from build123d import *

# Parameters (mm, degrees)
SKETCH2_W            = 38
SKETCH2_H            = 23.6
BOSS_EXTRUDE2_DEPTH  = 2.5
SKETCH3_W            = 35
SKETCH3_H            = 17.6
CUT_EXTRUDE2_DEPTH   = 2.5
SKETCH5_W            = 36.5
SKETCH5_H            = 2
SKETCH5_W_2          = 1.5
SKETCH5_H_2          = 19.6
BOSS_EXTRUDE3_DEPTH  = 26
SKETCH7_W            = 36.5
SKETCH7_H            = 2.5
BOSS_EXTRUDE5_DEPTH  = 1
SKETCH10_W           = 12.597499818
SKETCH10_H           = 2.5
SKETCH10_W_2         = 23.902500182
BOSS_EXTRUDE6_DEPTH  = 1
SKETCH11_W           = 2.5
SKETCH11_H           = 17.6
BOSS_EXTRUDE7_DEPTH  = 2
SKETCH15_W           = 30.589508609
SKETCH15_H           = 23.5
SKETCH15_W_2         = 3.8732763
CUT_EXTRUDE4_DEPTH   = 30
SKETCH16_W           = 3
SKETCH16_H           = 2.5
BOSS_EXTRUDE8_DEPTH  = 20
SKETCH17_W           = 3
SKETCH17_H           = 2.5
BOSS_EXTRUDE9_DEPTH  = 20
SKETCH19_W           = 5.5
SKETCH19_H           = 23.6
BOSS_EXTRUDE10_DEPTH = 16
SKETCH20_R           = 2.6
CUT_EXTRUDE6_DEPTH   = 30
SKETCH21_R           = 3.3
CUT_EXTRUDE7_DEPTH   = 0.8
SKETCH22_R           = 3.3
CUT_EXTRUDE8_DEPTH   = 0.8
FILLET1_R            = 5
FILLET3_R            = 5
SKETCH23_W           = 34.462784909
SKETCH23_H           = 2
BOSS_EXTRUDE11_DEPTH = 0.8
SKETCH24_W           = 34.462784909
SKETCH24_H           = 2
BOSS_EXTRUDE12_DEPTH = 0.8
SKETCH25_W           = 34.462784909
SKETCH25_H           = 2
BOSS_EXTRUDE13_DEPTH = 0.8
SKETCH26_W           = 34.462784909
SKETCH26_H           = 2
BOSS_EXTRUDE14_DEPTH = 0.8


with BuildPart() as part:
    # Sketch2 → Boss-Extrude2 (new body)
    with BuildSketch(Plane.XY):
        with Locations((19, 11.8)):
            Rectangle(SKETCH2_W, SKETCH2_H)
    extrude(amount=BOSS_EXTRUDE2_DEPTH)

    # Sketch3 → Cut-Extrude2 (cut)
    with BuildSketch(Plane.XY.offset(2.5)):
        with Locations((20.5, 11.8)):
            Rectangle(SKETCH3_W, SKETCH3_H)
    extrude(amount=-CUT_EXTRUDE2_DEPTH, mode=Mode.SUBTRACT)

    # Sketch5 → Boss-Extrude3 (add)
    with BuildSketch(Plane.XY.offset(2.5)):
        with Locations((19.75, 22.6)):
            Rectangle(SKETCH5_W, SKETCH5_H)
        with Locations((0.75, 22.6)):
            Rectangle(SKETCH5_W_2, SKETCH5_H)
        with Locations((0.75, 11.8)):
            Rectangle(SKETCH5_W_2, SKETCH5_H_2)
        with Locations((0.75, 1)):
            Rectangle(SKETCH5_W_2, SKETCH5_H)
        with Locations((19.75, 1)):
            Rectangle(SKETCH5_W, SKETCH5_H)
    extrude(amount=BOSS_EXTRUDE3_DEPTH)

    # Sketch7 → Boss-Extrude5 (add)
    with BuildSketch(Plane(origin=(0, 2, 0), x_dir=(1, 0, 0), z_dir=(0, 1, 0))):
        with Locations((19.75, -27.25)):
            Rectangle(SKETCH7_W, SKETCH7_H)
    extrude(amount=BOSS_EXTRUDE5_DEPTH)

    # Sketch10 → Boss-Extrude6 (add)
    with BuildSketch(Plane.XZ.offset(-21.6)):
        with Locations((31.701250091, 27.25)):
            Rectangle(SKETCH10_W, SKETCH10_H)
        with Locations((13.451250091, 27.25)):
            Rectangle(SKETCH10_W_2, SKETCH10_H)
    extrude(amount=BOSS_EXTRUDE6_DEPTH)

    # Sketch11 → Boss-Extrude7 (add)
    with BuildSketch(Plane(origin=(1.5, 0, 0), x_dir=(0, 0, -1), z_dir=(1, 0, 0))):
        with Locations((-27.25, 11.8)):
            Rectangle(SKETCH11_W, SKETCH11_H)
    extrude(amount=BOSS_EXTRUDE7_DEPTH)

    # Sketch15 → Cut-Extrude4 (cut)
    with BuildSketch(Plane(origin=(0, 23.6, 0), x_dir=(1, 0, 0), z_dir=(0, 1, 0))):
        with Locations((18.831969395, -14.25)):
            Rectangle(SKETCH15_W, SKETCH15_H)
        with Locations((36.06336185, -14.25)):
            Rectangle(SKETCH15_W_2, SKETCH15_H)
    extrude(amount=-CUT_EXTRUDE4_DEPTH, mode=Mode.SUBTRACT)

    # Sketch16 → Boss-Extrude8 (add)
    with BuildSketch(Plane(origin=(0, 3, 0), x_dir=(1, 0, 0), z_dir=(0, 1, 0))):
        with Locations((36.5, -1.25)):
            Rectangle(SKETCH16_W, SKETCH16_H)
    extrude(amount=BOSS_EXTRUDE8_DEPTH)

    # Sketch17 → Boss-Extrude9 (add)
    with BuildSketch(Plane(origin=(0, 3, 0), x_dir=(1, 0, 0), z_dir=(0, 1, 0))):
        with Locations((36.5, -27.25)):
            Rectangle(SKETCH17_W, SKETCH17_H)
    extrude(amount=BOSS_EXTRUDE9_DEPTH)

    # Sketch19 → Boss-Extrude10 (add)
    with BuildSketch(Plane.ZY):
        with Locations((17, 11.8)):
            Rectangle(SKETCH19_W, SKETCH19_H)
        with Locations((11.5, 11.8)):
            Rectangle(SKETCH19_W, SKETCH19_H)
    extrude(amount=BOSS_EXTRUDE10_DEPTH)

    # Sketch20 → Cut-Extrude6 (cut)
    with BuildSketch(Plane(origin=(0, 23.6, 0), x_dir=(1, 0, 0), z_dir=(0, 1, 0))):
        with Locations((-8.54, -14.25)):
            Circle(SKETCH20_R)
    extrude(amount=-CUT_EXTRUDE6_DEPTH, mode=Mode.SUBTRACT)

    # Sketch21 → Cut-Extrude7 (cut)
    with BuildSketch(Plane(origin=(0, 23.6, 0), x_dir=(1, 0, 0), z_dir=(0, 1, 0))):
        with Locations((-8.54, -14.25)):
            Circle(SKETCH21_R)
    extrude(amount=-CUT_EXTRUDE7_DEPTH, mode=Mode.SUBTRACT)

    # Sketch22 → Cut-Extrude8 (cut)
    with BuildSketch(Plane.XZ):
        with Locations((-8.54, 14.25)):
            Circle(SKETCH22_R)
    extrude(amount=-CUT_EXTRUDE8_DEPTH, mode=Mode.SUBTRACT)

    # Fillet1
    fillet1_edges = [part.edges().sort_by_distance(p)[0] for p in [
        (-16, 11.8, 8.75),
    ]]
    fillet(fillet1_edges, radius=FILLET1_R)

    # Fillet3
    fillet3_edges = [part.edges().sort_by_distance(p)[0] for p in [
        (-16, 11.8, 19.75),
    ]]
    fillet(fillet3_edges, radius=FILLET3_R)

    # Sketch23 → Boss-Extrude11 (add)
    with BuildSketch(Plane(origin=(0, 0, 26), x_dir=(-1, 0, 0), z_dir=(0, 0, -1))):
        with Locations((-20.768607546, 22.6)):
            Rectangle(SKETCH23_W, SKETCH23_H)
    extrude(amount=BOSS_EXTRUDE11_DEPTH)

    # Sketch24 → Boss-Extrude12 (add)
    with BuildSketch(Plane.XY.offset(2.5)):
        with Locations((20.768607546, 22.6)):
            Rectangle(SKETCH24_W, SKETCH24_H)
    extrude(amount=BOSS_EXTRUDE12_DEPTH)

    # Sketch25 → Boss-Extrude13 (add)
    with BuildSketch(Plane(origin=(0, 0, 26), x_dir=(-1, 0, 0), z_dir=(0, 0, -1))):
        with Locations((-20.768607546, 1)):
            Rectangle(SKETCH25_W, SKETCH25_H)
    extrude(amount=BOSS_EXTRUDE13_DEPTH)

    # Sketch26 → Boss-Extrude14 (add)
    with BuildSketch(Plane.XY.offset(2.5)):
        with Locations((20.768607546, 1)):
            Rectangle(SKETCH26_W, SKETCH26_H)
    extrude(amount=BOSS_EXTRUDE14_DEPTH)


solid = part.part
Here's how the part is built. I have some questions about the finished solid (model axes, mm). A direction names the side the tool comes from. Round coordinates to 2 decimals unless told otherwise and drop trailing zeros. Order: outer loops, then holes, each group sorted by start corner. A loop starts at its lowest first (then second) coordinate and runs counter-clockwise, first axis right, second up. Notation, with made-up numbers: (40.25, 77) -> (81.25, 77) arc R14 cw to (81.25, 98) -> close; hole circle Ø7 at (75.25, -10). An arc over 180 degrees is marked (long way). Use CSV: the item, a comma, the result in double quotes.
1. I want a section at D-D on z = 4.5. List the corners of the cut face in (x, y) for me.
Recorded:
outline,"(0, 0) -> (3.54, 0) -> (3.54, 2) -> (1.5, 2) -> (1.5, 21.6) -> (3.54, 21.6) -> (3.54, 23.6) -> (0, 23.6) -> close"
2. I'm going to push flat-ended pins straight in: P1, Ø7, axis at y = 12, z = 3, coming from the -X side; P2, Ø2, axis at x = -10, z = 13.5, coming from the +Y side; P3, Ø6, axis at y = 20, z = 8, coming from the -X side; P4, Ø4, axis at x = 24, y = 6, coming from the -Z side. Where does each tip first touch, or does it pass through?
Recorded:
P1,"stops at x = 0"
P2,"stops at y = 22.8"
P3,"stops at x = -15.18"
P4,"passes through"
3. I want a section at C-C on x = -8.54. List the corners of the cut face in (y, z) for me.
Recorded:
outline,"(0, 8.75) -> (23.6, 8.75) -> (23.6, 10.95) -> (22.8, 10.95) -> (22.8, 11.65) -> (0.8, 11.65) -> (0.8, 10.95) -> (0, 10.95) -> close; (0, 17.55) -> (0.8, 17.55) -> (0.8, 16.85) -> (22.8, 16.85) -> (22.8, 17.55) -> (23.6, 17.55) -> (23.6, 19.75) -> (0, 19.75) -> close"
4. Thinking about a two-plate mould opening in Z: for faces 6 (the face through (19, 3, 1)), 7 (the face through (19, 22, 0)), 8 (the face through (24, 21, 2.5)), 9 (the face through (-14.57, 11.97, 18.25)), which applies, pulls with the +Z half, pulls with the -Z half, needs draft (parallel to the pull), parting line crosses it, or undercut?
Recorded:
face 6,"needs draft"
face 7,"pulls with the -Z half"
face 8,"undercut"
face 9,"pulls with the +Z half"
5. I want a section at B-B on x = 34. List the corners of the cut face in (y, z) for me.
Recorded:
outline,"(0, 0) -> (3, 0) -> (3, 2.5) -> (2, 2.5) -> (2, 3.3) -> (0, 3.3) -> close; (0, 25.2) -> (2, 25.2) -> (2, 26) -> (3, 26) -> (3, 28.5) -> (0, 28.5) -> close; (20.6, 0) -> (23.6, 0) -> (23.6, 3.3) -> (21.6, 3.3) -> (21.6, 2.5) -> (20.6, 2.5) -> close; (20.6, 26) -> (21.6, 26) -> (21.6, 25.2) -> (23.6, 25.2) -> (23.6, 28.5) -> (20.6, 28.5) -> close"
6. I need wall thicknesses on line 1 along Z through (x, y) = (-8.54, 10); line 2 along Y through (x, z) = (17.5, 26.25); line 3 along Y through (x, z) = (3.5, 10). Which ranges of each line are inside material? Lowest first, please.
Recorded:
line 1,"z = 8.75 to 11.65, 16.85 to 19.75"
line 2,"y = 0 to 3, 20.6 to 23.6"
line 3,"y = 0 to 2, 21.6 to 23.6"
7. Which directions (+Z, -Z, +X, -X, +Y, -Y) give clear straight access to the entire face, cutting with the end or side of a thin tool? Please do faces 1 (the face through (-5, 12, 8.75)), 2 (the face through (1.5, 12, 14)), 3 (the face through (21, 1, 25.2)), 4 (the face through (19, 20.6, 27)), 5 (the face through (-5, 12, 19.75)).
Recorded:
face 1,"-Z, -X, +Y, -Y"
face 2,"+X"
face 3,"+X, +Y, -Y"
face 4,"+Z, -Z"
face 5,"+Z, -X, +Y, -Y"
8. I want a section at A-A on y = 5.75. List the corners of the cut face in (x, z) for me, and give its area (3 significant figures).
Recorded:
outline,"(-16, 13.75) arc R5 ccw to (-11, 8.75) -> (0, 8.75) -> (0, 0) -> (3, 0) -> (3, 2.5) -> (1.5, 2.5) -> (1.5, 26) -> (3.5, 26) -> (3.5, 28.5) -> (0, 28.5) -> (0, 19.75) -> (-11, 19.75) arc R5 ccw to (-16, 14.75) -> close; (35, 0) -> (38, 0) -> (38, 2.5) -> (35, 2.5) -> close; (35, 26) -> (38, 26) -> (38, 28.5) -> (35, 28.5) -> close; hole circle Ø5.2 at (-8.54, 14.25)"
area,"211 mm2"
